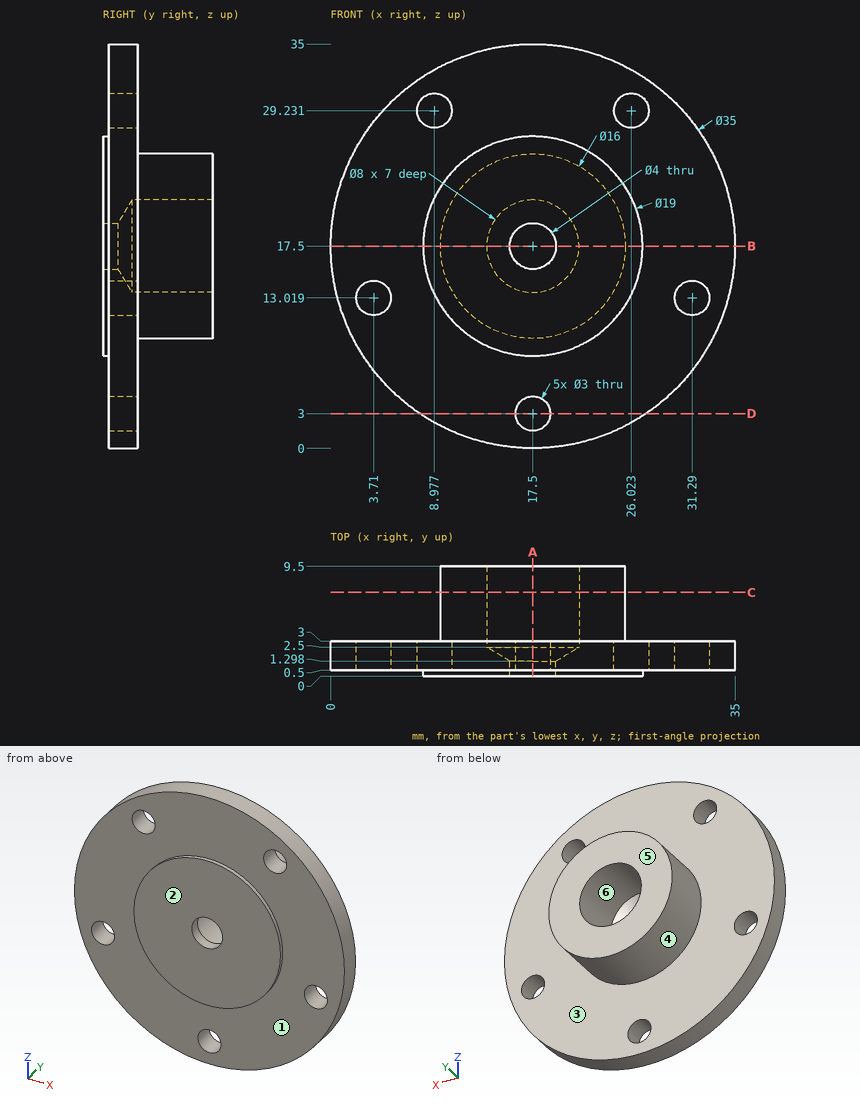
Input: dimensioned drawing with shaded views. Units: mm. Origin: part minimum x, y, z. A direction names the side the tool comes from. Give positions to 0.01 mm unless a question says otherwise; leave off trailing zeros. Loops run counter-clockwise (first coordinate to the right, second up) from the corner with the lowest first, then second, coordinate; pieces in that order, holes last. Notation, with made-up numbers: M -31.75,-4 L -23.75,-4 A22 cw -23.75,32 Z; hole C 17.5,29.5 d2. An arc over 180 degrees is marked long. Put each result on its own line as item: value. Start each with the question number.
1) Cut plane A-A (x = 17.5). Output: boundary loops of the cut face in (y, z), then the cut area to 3 significant figures.
2) Cut plane C-C (y = 7.25). Output: boundary loops of the cut face in (x, z).
3) Pull-direction query (X, two-part tool) for the marked faces 4, 5 and 6; classes: pulls with the +X half, pulls with the -X half, needs draft (parallel to the pull), parting line crosses it, or undercut.
4) Access query for the marked faces 1, 2 and 3. Directions: +Z, -Z, +X, -X, +Y, -Y. A direction counts if a zero-diameter tool reaches every point of the face in a straight line with its end or side. Return the directions, or none.
5) Cut plane D-D (z = 3). Output: boundary loops of the cut face in (x, y), then the cut area to 3 significant figures.
6) Cut plane B-B (z = 17.5). Output: boundary loops of the cut face in (x, y), then the cut area to 3 significant figures.
7) Contact query for flat-ended pins moving along their axis: pin 1 (5 mm diameter, centred on x = 31.29, z = 13.02, fed in from -Y); pin 2 (4 mm diameter, centred on x = 25.5, y = 8, fed in from +Z); pin 3 (3 mm diameter, centred on x = 28.5, z = 10.5, fed in from +Y). Output: stop coordinate, or through.
8) Ray query, line 1 along Z through (x, y) = (17.5, 4.5); line 2 along X through (y, z) = (2.25, 13.5); line 3 along Y through (x, z) = (8, 11.5). Return the intervals inside material, ascending.
Verdict:
1. outline: M 0,8 L 0.5,8 L 0.5,4.5 L 3,4.5 L 3,9.5 L 9.5,9.5 L 9.5,13.5 L 2.5,13.5 L 1.3,15.5 L 0,15.5 Z; M 0,19.5 L 1.3,19.5 L 2.5,21.5 L 9.5,21.5 L 9.5,25.5 L 3,25.5 L 3,35 L 0.5,35 L 0.5,27 L 0,27 Z; M 0.5,0 L 3,0 L 3,1.5 L 0.5,1.5 Z
1. area: 125 mm2
2. outline: C 17.5,17.5 d16; hole C 17.5,17.5 d8
3. face 4: parting line crosses it
3. face 5: needs draft
3. face 6: undercut
4. face 1: -Y
4. face 2: +Z, -Z, +X, -X, -Y
4. face 3: +Y
5. outline: M 7.7,0.5 L 16,0.5 L 16,3 L 7.7,3 Z; M 19,0.5 L 27.3,0.5 L 27.3,3 L 19,3 Z
5. area: 41.5 mm2
6. outline: M 0,0.5 L 8,0.5 L 8,0 L 15.5,0 L 15.5,1.3 L 13.5,2.5 L 13.5,9.5 L 9.5,9.5 L 9.5,3 L 0,3 Z; M 19.5,0 L 27,0 L 27,0.5 L 35,0.5 L 35,3 L 25.5,3 L 25.5,9.5 L 21.5,9.5 L 21.5,2.5 L 19.5,1.3 Z
6. area: 133 mm2
7. pin 1: y = 0.5
7. pin 2: z = 22.79
7. pin 3: y = 3
8. line 1: 9.5 to 13.5, 21.5 to 25.5
8. line 2: 0.46 to 2.29, 5.13 to 29.87, 32.71 to 34.54
8. line 3: 0.5 to 3
